Part print with two shaded views. Sizes in mm from the minimum x, y, z corner. A direction names the side the tool comes from. Coordinates: 2 decimals unless noted, no trailing zeros. Loops run counter-clockwise (first coordinate to the right, second up) from the corner with the lowest first, then second, coordinate; pieces in that order, holes last.
(1) Flat gauge pins, fed straight in: P1, Ø3, axis at y = 4.5, z = 9.5, coming from the +X side; P2, Ø1, axis at y = 2.5, z = 5, coming from the -X side (3 decimals); P3, Ø1.5, axis at y = 1.5, z = 4.5, coming from the +X side. Where does each tip first touch, or does it go through?
(2) Slice it at B-B (z = 4). Give the cut face in (x, y) (1 decimal).
(3) Slice it at C-C (z = 10). Give the cut face in (x, y) (1 decimal).
(4) Tool access for the marked faces 3 and 4: list every direction of +Z, -Z, +X, -X, +Y, -Y with a clear straight run to the whole face (end or side of a thin tool).
(5) Slice it at A-A (y = 2.8). Give the cut face in (x, z) (1 decimal).
(6) Wall check: L1, parallel to X at y = 2.9, z = 3.75; L2, parallel to Y at x = 2.8, z = 6.5; L3, parallel to Y at x = 3.85, z = 2.5. Give the ranges that are in metal, low to high.
(7) Two-plate mould, pull along X, no slides. Class the marked faces 1 and 2: pulls with the +X half, pulls with the -X half, needs draft (parallel to the pull), parting line crosses it, or undercut.
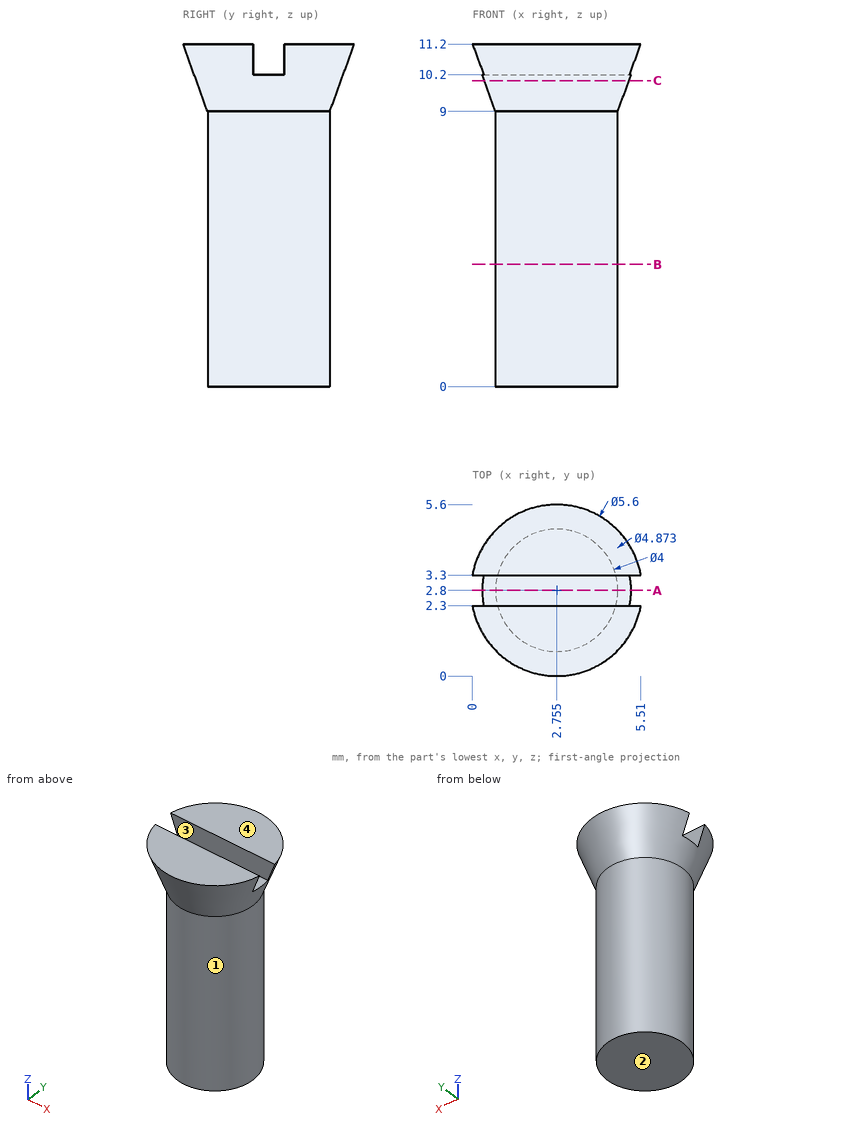
Response values:
1. P1: stops at x = 5.25
1. P2: stops at x = 0.755
1. P3: stops at x = 4.68
2. outline: circle Ø4 at (2.8, 2.8)
3. outline: circle Ø4.7 at (2.8, 2.8)
4. face 3: +Z, +X, -X
4. face 4: +Z, +X, -X, +Y, -Y
5. outline: (0.3, 10.2) - (0.8, 9) - (0.8, 0) - (4.8, 0) - (4.8, 9) - (5.2, 10.2) - close
6. L1: x = 0.76 to 4.75
6. L2: y = 0.8 to 4.8
6. L3: y = 1.13 to 4.47
7. face 1: parting line crosses it
7. face 2: needs draft
